```python
from build123d import *

# Parameters (mm, degrees)
SKETCH5_R           = 12.7
BOSS_EXTRUDE4_DEPTH = 3.175


with BuildPart() as part:
    # Sketch5 → Boss-Extrude4 (new body)
    with BuildSketch(Plane.XY):
        Polygon((0, 35.56), (0, 0), (203.2, 0), (203.2, -93.533944169), (372.637377726, -93.533944169), (267.345580387, -42.014632685), (270.136458661, -36.310818307), (387.085338563, -93.533944169), (558.8, -93.533944169), (558.8, 35.56), align=None)
        with Locations((231.775, -58.608944169)):
            Circle(SKETCH5_R, mode=Mode.SUBTRACT)
        Polygon((25.06325275, 24.691281209), (25.711364465, 11.991281209), (15.036897694, 5.08), (3.714319208, 10.868718791), (3.066207494, 23.568718791), (13.740674265, 30.48), align=None, mode=Mode.SUBTRACT)
        with Locations((511.175, -20.248310315)):
            Circle(SKETCH5_R, mode=Mode.SUBTRACT)
    extrude(amount=BOSS_EXTRUDE4_DEPTH)


solid = part.part
```
Model file for the job. Use its own axes, mm. A direction names the side the tool comes from. Coordinates: 2 decimals unless noted, no trailing zeros. Order: outer loops, then holes, each group sorted by start corner. A loop starts at its lowest first (then second) coordinate and runs counter-clockwise, first axis right, second up. Notation, with made-up numbers: (-30, -11) - (-24, -11) arc R23 ccw to (-24, 3) - close; hole circle Ø1 at (41.5, 81.25). An arc over 180 degrees is marked (long way). Return JSON: item names as keys, results as strings. Group by question number.
1) Saw through at C-C, the plane z = 1.6. Write the cut outline in (x, y) (3 decimals).
2) Flat gauge pins, fed straight in: P1, Ø15, axis at x = 231.78, y = -58.61, coming from the +Z side; P2, Ø1, axis at y = -23, z = 0.5, coming from the -X side. Where does each tip first touch, or does it go through?
3) Saw through at D-D, the plane y = 17.5. Write the cut outline in (x, z) (3 decimals), plus the area to 3 significant figures.
4) Mould opens along X. For faces 3 (the flat face through (338, -14, 3.175)), 4 (the flat face through (320.729, -68.135, 1.565)) say: released by +X, released by -X, zero draft, split by the parting line, or undercut.
5) Tool access for faces 1 (the flat face through (338, -14, 0)), 2 (the flat face through (327.79, -64.52, 1.57)): list every direction of +Z, -Z, +X, -X, +Y, -Y with a clear straight run to the whole face (end or side of a thin tool).
6) Saw through at B-B, the plane x = 312.5. Write the cut outline in (y, z) (3 decimals), plus the area to 3 significant figures.
7) Probe line 1 (X direction, y = -49, z = 1.5); line 2 (X direction, y = -62.5, z = 3); line 3 (Y direction, x = 148, z = 1.65). List the from-to ranges inside material, lowest first. Write a range as from..to.
8) Saw through at A-A, the plane y = -51.5. Write the cut outline in (x, z) (3 decimals).
Values found:
{
 "1": {"outline": "(0, 0) - (203.2, 0) - (203.2, -93.534) - (372.637, -93.534) - (267.346, -42.015) - (270.136, -36.311) - (387.085, -93.534) - (558.8, -93.534) - (558.8, 35.56) - (0, 35.56) - close; hole (3.066, 23.569) - (3.714, 10.869) - (15.037, 5.08) - (25.711, 11.991) - (25.063, 24.691) - (13.741, 30.48) - close; hole circle Ø25.4 at (231.775, -58.609); hole circle Ø25.4 at (511.175, -20.248)"},
 "2": {"P1": "passes through", "P2": "stops at x = 203.2"},
 "3": {"outline": "(0, 0) - (3.376, 0) - (3.376, 3.175) - (0, 3.175) - close; (25.43, 0) - (558.8, 0) - (558.8, 3.175) - (25.43, 3.175) - close", "area": "1,700 mm²"},
 "4": {"face 3": "zero draft", "face 4": "undercut"},
 "5": {"face 1": "-Z, +X, -X, +Y, -Y", "face 2": "+Z, -Z"},
 "6": {"outline": "(-93.534, 0) - (-64.109, 0) - (-64.109, 3.175) - (-93.534, 3.175) - close; (-57.039, 0) - (35.56, 0) - (35.56, 3.175) - (-57.039, 3.175) - close", "area": "387 mm²"},
 "7": {"line 1": "x = 203.2..223.47, 240.08..281.62, 296.07..558.8", "line 2": "x = 203.2..219.69, 243.86..309.21, 323.66..558.8", "line 3": "y = 0..35.56"},
 "8": {"outline": "(203.2, 0) - (221.251, 0) - (221.251, 3.175) - (203.2, 3.175) - close; (242.299, 0) - (286.731, 0) - (286.731, 3.175) - (242.299, 3.175) - close; (301.179, 0) - (558.8, 0) - (558.8, 3.175) - (301.179, 3.175) - close"}
}
